Source: three-view drawing plus pictorial views. Frame: mm from the lowest corner of the part. Coordinates: 2 decimals unless noted, no trailing zeros. Order: outer loops, then holes, each group sorted by start corner. A loop starts at its lowest first (then second) coordinate and runs counter-clockwise, first axis right, second up. Notation, with made-up numbers: M 65.5,35.5 L 83.5,35.5 A35 ccw 83.5,68.5 Z; hole C 41,49.25 d4. An arc over 180 degrees is marked long. Write item = value, one per line. Start each with the question number.
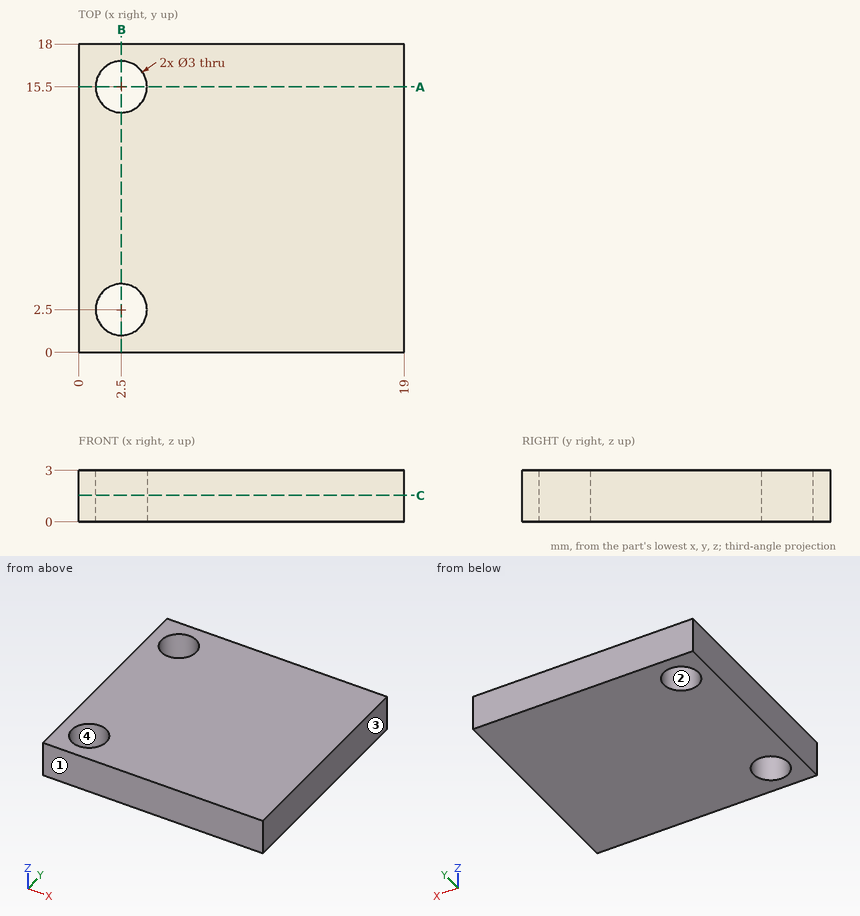
Item 1: Section query B-B on x = 2.5. Output: boundary loops of the cut face in (y, z), and give its area (3 significant figures).
Item 2: Section query A-A on y = 15.5. Output: boundary loops of the cut face in (x, z).
Item 3: Material intervals for probe 1 along Y at (x, z) = (2.5, 1.7); probe 2 along Y at (x, z) = (1.5, 2.25); probe 3 along X at (y, z) = (16.25, 0.95), sorted ascending. Write a range as [from, to].
Item 4: Section query C-C on z = 1.55. Output: boundary loops of the cut face in (x, y).
Item 5: Draft query along Y for the marked faces 1, 2, 3 and 4. Return one class per face: pulls with the +Y half, pulls with the -Y half, needs draft (parallel to the pull), parting line crosses it, or undercut.
Ans:
q1.outline = M 0,0 L 1,0 L 1,3 L 0,3 Z; M 4,0 L 14,0 L 14,3 L 4,3 Z; M 17,0 L 18,0 L 18,3 L 17,3 Z
q1.area = 36.0 mm^2
q2.outline = M 0,0 L 1,0 L 1,3 L 0,3 Z; M 4,0 L 19,0 L 19,3 L 4,3 Z
q3.probe_1 = [0, 1], [4, 14], [17, 18]
q3.probe_2 = [0, 1.38], [3.62, 14.38], [16.62, 18]
q3.probe_3 = [0, 1.2], [3.8, 19]
q4.outline = M 0,0 L 19,0 L 19,18 L 0,18 Z; hole C 2.5,2.5 d3; hole C 2.5,15.5 d3
q5.face_1 = pulls with the -Y half
q5.face_2 = undercut
q5.face_3 = needs draft
q5.face_4 = undercut
